Part print with two shaded views. Sizes in mm from the minimum x, y, z corner. Round coordinates to 2 decimals unless told otherwise and drop trailing zeros. Write each loop counter-clockwise with the first axis right and the second up, starting at its lowest first coordinate (ties: lowest second). Pieces come first, ordered by that corner, then holes. Notation, with made-up numbers: (29, 71) -> (35, 71) arc R19 cw to (35, 75) -> close; hole circle Ø8 at (-4.5, 20.5). An arc over 180 degrees is marked (long way). Answer in a Markdown table with one row per item.
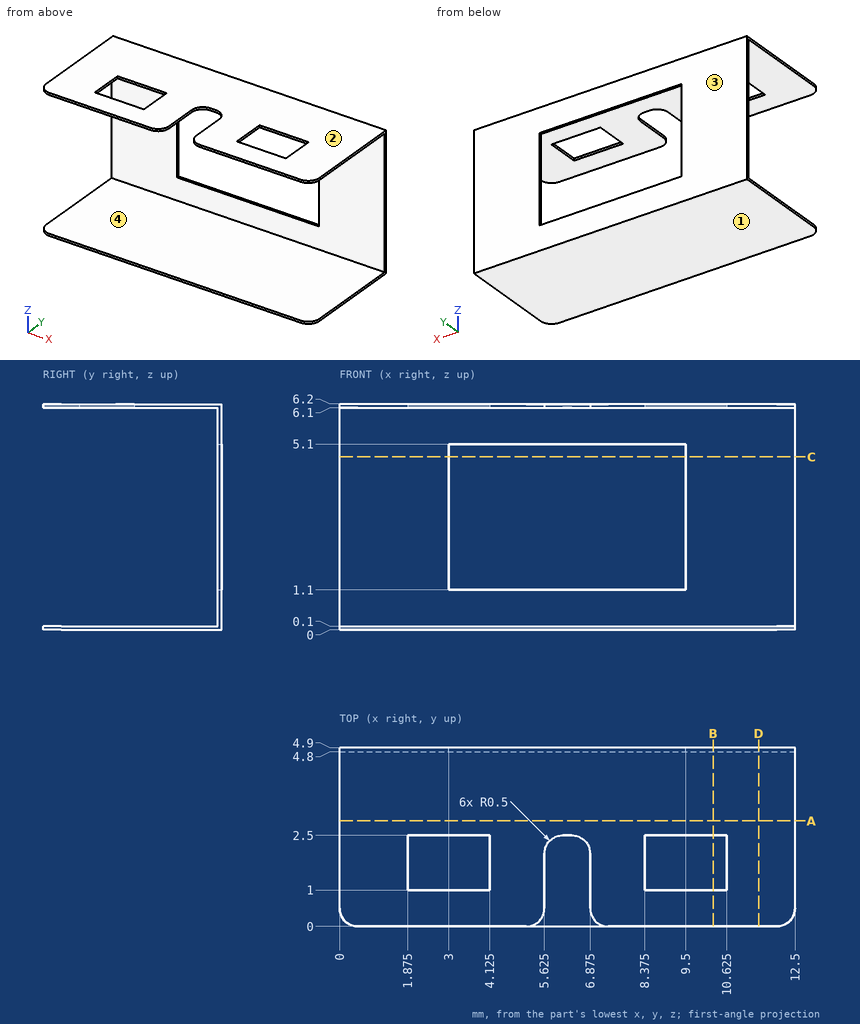
Q1. Two-plate mould, pull along Z, no slides. Class the marked faces 1, 2, 3 and 4: released by +Z, released by -Z, zero draft, split by the parting line, or undercut.
A:
| item | result |
|---|---|
| face 1 | released by -Z |
| face 2 | released by +Z |
| face 3 | zero draft |
| face 4 | undercut |
Q2. Drop a flat-ended pin along its axis: P1, Ø1, axis at y = 2.5, z = 5.5, coming from the -X side. Give the stop position or say it passes through.
A:
| item | result |
|---|---|
| P1 | through |
Q3. Saw through at C-C on z = 4.75. Write the cut outline in (x, y), plus the area to 3 significant figures.
A:
| item | result |
|---|---|
| outline | (0, 4.8) -> (3, 4.8) -> (3, 4.9) -> (0, 4.9) -> close; (9.5, 4.8) -> (12.5, 4.8) -> (12.5, 4.9) -> (9.5, 4.9) -> close |
| area | 0.600 mm² |
Q4. Saw through at B-B on x = 10.25. Write the cut outline in (y, z).
A:
| item | result |
|---|---|
| outline | (0, 0) -> (4.9, 0) -> (4.9, 6.2) -> (2.5, 6.2) -> (2.5, 6.1) -> (4.8, 6.1) -> (4.8, 0.1) -> (0, 0.1) -> close; (0, 6.1) -> (1, 6.1) -> (1, 6.2) -> (0, 6.2) -> close |
Q5. Saw through at A-A on y = 2.9. Write the cut outline in (x, z).
A:
| item | result |
|---|---|
| outline | (0, 0) -> (12.5, 0) -> (12.5, 0.1) -> (0, 0.1) -> close; (0, 6.1) -> (12.5, 6.1) -> (12.5, 6.2) -> (0, 6.2) -> close |
Q6. Saw through at D-D on x = 11.5. Write the cut outline in (y, z), plus the area to 3 significant figures.
A:
| item | result |
|---|---|
| outline | (0, 0) -> (4.9, 0) -> (4.9, 6.2) -> (0, 6.2) -> (0, 6.1) -> (4.8, 6.1) -> (4.8, 0.1) -> (0, 0.1) -> close |
| area | 1.58 mm² |
